Work out the finished part from the listing and answer in its coordinate system (mm). Face numbers are marked on the shaded views. A direction names the side the tool comes from. Give positions to 0.01 mm unless a question says otherwise; leave off trailing zeros. Write each loop counter-clockwise with the first axis right and the second up, starting at its lowest first coordinate (ties: lowest second). Pieces come first, ordered by that corner, then holes. Notation, with made-up numbers: (45.5, 29.25) -> (102.5, 29.25) arc R23 ccw to (102.5, 44.25) -> close; hole circle Ø4 at (36, -6.75). An arc over 180 degrees is marked (long way). Use a Markdown table: item, result. Add a question column.
Q1. Section D-D, the plane x = -38 is taken. Give the vertices of the cut face in (y, z), plus the area to 3 significant figures.
Q2. Section A-A, the plane x = 0 is taken. Give the vertices of the cut face in (y, z).
Q3. For the marked faces 4, 5 and 6, determine the directions among +Z, -Z, +X, -X, +Y, -Y from which every point of the face is accessible in a straight line to the end or side of a thin tool.
Q4. For a pull along Y with two mould halves and no side action, classify the marked faces 1, 2 and 3 as pulls with the +Y half, pulls with the -Y half, needs draft (parallel to the pull), parting line crosses it, or undercut.
Q5. Each of these flat-tipped pins is pushed along its axis until it touches: pin 1 Ø2 at (x, z) = (7, 128.5) entering from +Y; pin 2 Ø8 at (x, y) = (-49, 0) entering from -Z; pin 3 Ø12 at (x, z) = (-26.5, 127.5) entering from +Y. Where does it stop, or does it pass through?
Q6. Section C-C, the plane z = 37 is taken. Give the vertices of the cut face in (x, y) (3 decimals), plus the area to 3 significant figures.
Q7. Consider line 1 (Z direction, x = 30, y = -38); line 2 (Y direction, x = 34, z = 57.5); line 3 (X direction, y = -24, z = 113). Determine where each line is inside the solid, lowest interval first.
from build123d import *

# Parameters (mm, degrees)
SKETCH1_R           = 54.61
BOSS_EXTRUDE1_DEPTH = 170.18
BOSS_EXTRUDE2_START = -170.18
SKETCH2_R           = 6.35
BOSS_EXTRUDE2_DEPTH = 25.4
BOSS_EXTRUDE3_DEPTH = 63.5
SKETCH4_R           = 4.7625
SKETCH4_W           = 3.175
SKETCH4_H           = 63.5
BOSS_EXTRUDE4_DEPTH = 6.35


with BuildPart() as part:
    # Sketch1 → Boss-Extrude1 (new body)
    with BuildSketch(Plane.XY):
        Circle(SKETCH1_R)
    extrude(amount=BOSS_EXTRUDE1_DEPTH)

    # Sketch2 → Boss-Extrude2 (add)
    with BuildSketch(Plane.XY.offset(170.18).offset(BOSS_EXTRUDE2_START)):
        Circle(SKETCH2_R)
    extrude(amount=-BOSS_EXTRUDE2_DEPTH)

    # Sketch3 → Boss-Extrude3 (add)
    with BuildSketch(Plane.XY):
        with BuildLine():
            Line((-31.288001325, -44.758385506), (-44.314615818, -57.785))
            Line((-44.314615818, -57.785), (-47.489615818, -57.785))
            Line((-47.489615818, -57.785), (-47.489615818, -64.135))
            Line((-47.489615818, -64.135), (-41.928035591, -64.135))
            Line((-41.928035591, -64.135), (-25.880821668, -48.087786077))
            ThreePointArc((-25.880821668, -48.087786077), (-28.63284491, -46.501745047), (-31.288001325, -44.758385506))
        make_face()
    extrude(amount=BOSS_EXTRUDE3_DEPTH)

    # Sketch4 → Boss-Extrude4 (add)
    # profile 1 of 2: a face of its own
    with BuildSketch(Plane(origin=(0, -57.785, 0), x_dir=(1, 0, 0), z_dir=(0, 1, 0))):
        Polygon((-72.889615818, -73.025), (-53.839615818, -73.025), (-44.314615818, -63.5), (-47.489615818, -63.5), (-47.489615818, 0), (-44.314615818, 0), (-53.839615818, 9.525), (-72.889615818, 9.525), align=None)
        with Locations(Location((-63.364615818, -63.5, 0), (0, 0, 180))):
            Circle(SKETCH4_R, mode=Mode.SUBTRACT)
        with Locations(Location((-63.364615818, 0, 0), (0, 0, 180))):
            Circle(SKETCH4_R, mode=Mode.SUBTRACT)
    # profile 2 of 2: a face of its own
    with BuildSketch(Plane(origin=(0, -57.785, 0), x_dir=(1, 0, 0), z_dir=(0, 1, 0))):
        with Locations((-45.902115818, -31.75)):
            Rectangle(SKETCH4_W, SKETCH4_H)
    extrude(amount=-BOSS_EXTRUDE4_DEPTH)

    # Mirror1: part across plane


with BuildPart() as part_1:
    add(part.part)
    add(part.part.mirror(Plane(origin=(0, 0, 0), x_dir=(0, 0, 1), z_dir=(1, 0, 0))))


solid = part_1.part
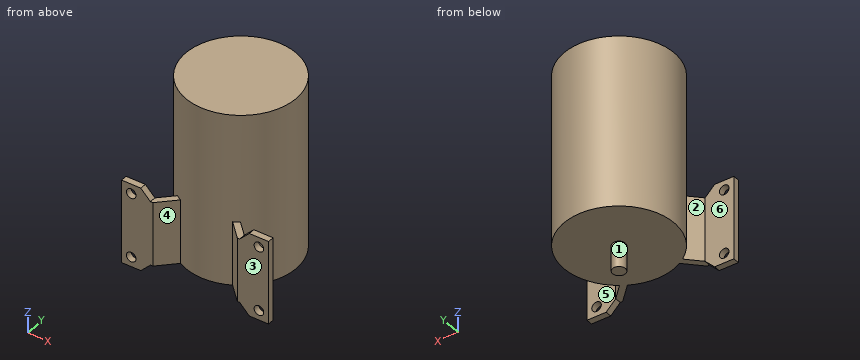
Result set:
| question | item | result |
|---|---|---|
| 1 | outline | (-60.21, 0) -> (-51.47, 0) -> (-51.47, 63.5) -> (-60.21, 63.5) -> close; (-39.22, 0) -> (39.22, 0) -> (39.22, 170.18) -> (-39.22, 170.18) -> close |
| 1 | area | 13,900 mm2 |
| 2 | outline | (-54.61, 0) -> (-6.35, 0) -> (-6.35, -25.4) -> (6.35, -25.4) -> (6.35, 0) -> (54.61, 0) -> (54.61, 170.18) -> (-54.61, 170.18) -> close |
| 3 | face 4 | +Z, -Z, -Y |
| 3 | face 5 | +Z, -Z, +X |
| 3 | face 6 | +Z, -Z, -X |
| 4 | face 1 | parting line crosses it |
| 4 | face 2 | undercut |
| 4 | face 3 | pulls with the -Y half |
| 5 | pin 1 | stops at y = 54.28 |
| 5 | pin 2 | stops at z = 0 |
| 5 | pin 3 | stops at y = 50.62 |
| 6 | outline | (-72.89, -64.135) -> (-41.928, -64.135) -> (-25.881, -48.088) arc R54.61 ccw to (25.881, -48.088) -> (41.928, -64.135) -> (72.89, -64.135) -> (72.89, -57.785) -> (44.315, -57.785) -> (31.288, -44.758) arc R54.61 ccw (long way) to (-31.288, -44.758) -> (-44.315, -57.785) -> (-72.89, -57.785) -> close |
| 6 | area | 10,000 mm2 |
| 7 | line 1 | z = 0 to 170.18 |
| 7 | line 2 | y = -56.21 to -47.47, -42.73 to 42.73 |
| 7 | line 3 | x = -49.05 to 49.05 |
